The drawing under review shows one solid part. Ordinate dimensions are in mm from its lowest x, y, z. A direction names the side the tool comes from. Give positions to 0.01 mm unless a question says otherwise; leave off trailing zeros. Loops run counter-clockwise (first coordinate to the right, second up) from the corner with the lowest first, then second, coordinate; pieces in that order, holes last.
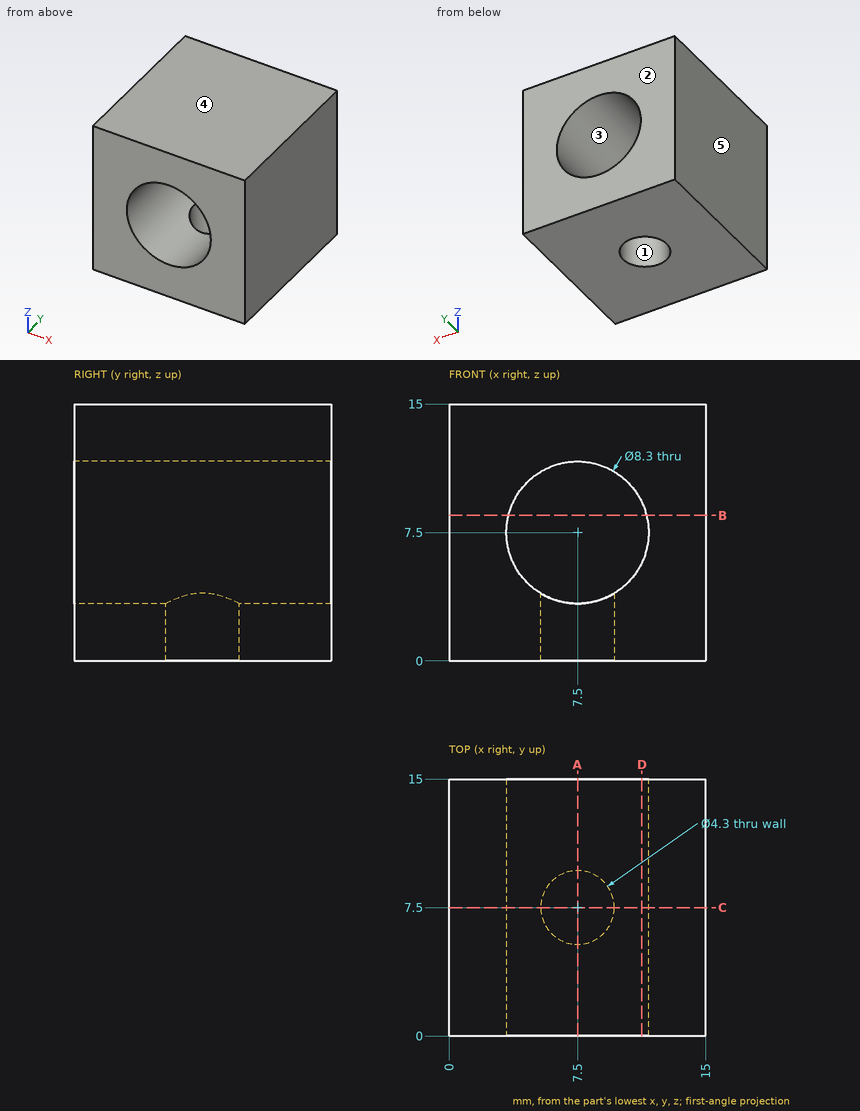
Item 1: Take a section at B-B on z = 8.5. Give the boundary of the cut face in (x, y).
Answer:
outline: (0, 0) - (3.47, 0) - (3.47, 15) - (0, 15) - close; (11.53, 0) - (15, 0) - (15, 15) - (11.53, 15) - close
Item 2: Take a section at A-A on x = 7.5. Give the boundary of the cut face in (y, z).
Answer:
outline: (0, 0) - (5.35, 0) - (5.35, 3.35) - (0, 3.35) - close; (0, 11.65) - (15, 11.65) - (15, 15) - (0, 15) - close; (9.65, 0) - (15, 0) - (15, 3.35) - (9.65, 3.35) - close
Item 3: Tool access review of the marked faces 1 and 2: name each direction out of +Z, -Z, +X, -X, +Y, -Y from which nothing blocks a thin tool from reaching the whole face with its end or side.
Answer:
face 1: -Z
face 2: +Z, -Z, +X, -X, +Y
Item 4: The part is to be moulded in two halves that separate along Z. For the marked faces 3, 4 and 5, say which applies: released by +Z, released by -Z, zero draft, split by the parting line, or undercut.
Answer:
face 3: undercut
face 4: released by +Z
face 5: zero draft
Item 5: Take a section at C-C on y = 7.5. Give the boundary of the cut face in (x, z).
Answer:
outline: (0, 0) - (5.35, 0) - (5.35, 3.95) arc R4.15 cw (long way) to (9.65, 3.95) - (9.65, 0) - (15, 0) - (15, 15) - (0, 15) - close
Item 6: For L1, parallel to Y at x = 7.5, z = 1.7; L2, parallel to Z at x = 7.5, y = 11; L3, parallel to Z at x = 7.5, y = 7, list the stretches that pass through material, from the lowest coordinate up.
Answer:
L1: y = 0 to 5.35, 9.65 to 15
L2: z = 0 to 3.35, 11.65 to 15
L3: z = 11.65 to 15
Item 7: Take a section at D-D on x = 11.25. Give the boundary of the cut face in (y, z).
Answer:
outline: (0, 0) - (15, 0) - (15, 5.72) - (0, 5.72) - close; (0, 9.28) - (15, 9.28) - (15, 15) - (0, 15) - close
